Autodesk Fusion 360 part; units mm, degrees
sketch "Sketch1" plane through (0, 0, 0) normal (0, 0, 1) x (1, 0, 0)
  line L0 (0, 44) -> (67, 44)
  line L1 (67, -44) -> (0, -44)
  line L2 (0, 0) -> (67, 0) construction
  line L3 (0, 44) -> (0, -44)
  line L4 (80.435, -13.435) -> (49.8701, -44)
  line L5 (80.435, 13.435) -> (49.8701, 44)
  arc A0 (80.435, -13.435) -> (80.435, 13.435) centre (67, 0) ccw
  dimension "d2" = 67
  dimension "d3" = 88
  dimension "d4" = 67
  dimension "d6" = 38
  dimension "d9" = 45
  dimension "d10" = 45
extrude "Extrude2" add sketch "Sketch1" along normal blind 10
sketch "Sketch5" plane through (0, 0, 10) normal (0, 0, 1) x (-1, 0, 0)
  line L0 (-49.8701, 44) -> (-80.435, 13.435)
  arc A0 (-80.435, 13.435) -> (-80.435, -13.435) centre (-67, 0) ccw
  line L1 (-80.435, -13.435) -> (-49.8701, -44)
  line L2 (-49.8701, -44) -> (0, -44)
  line L3 (0, -44) -> (0, 44)
  line L4 (0, 44) -> (-49.8701, 44)
  line L5 (0, -44) -> (13, -44)
  line L6 (13, -44) -> (13, -19)
  line L7 (13, -19) -> (19, -19)
  line L8 (19, 0) -> (0, 0) construction
  line L9 (0, 44) -> (13, 44)
  line L10 (13, 44) -> (13, 19)
  line L11 (13, 19) -> (19, 19)
  arc A1 (19, -19) -> (19, 19) centre (19, 0) ccw
  line L12 (0, -19) -> (-3, -19)
  line L13 (-3, -19) -> (-3, -5)
  line L14 (-3, -5) -> (-7, -5)
  line L15 (-7, -5) -> (-7, 0)
  line L16 (0, 19) -> (-3, 19)
  line L17 (-3, 19) -> (-3, 5)
  line L18 (-3, 5) -> (-7, 5)
  line L19 (-7, 5) -> (-7, 0)
  line L20 (0, -44) -> (0, -19)
  line L21 (0, 19) -> (0, 44)
  dimension "d15" = 13
  dimension "d16" = 38
  dimension "d17" = 6
  dimension "d18" = 3
  dimension "d19" = 14
  dimension "d20" = 4
extrude "Extrude4" add sketch "Sketch5" along normal blind 40 contours L3 L12 L13 L14 L15 L16 L17 L18 L19
extrude "Extrude3" add sketch "Sketch5" along normal blind 40 and the other way blind 10 contours L3 L5 L6 L7 L9 L10 L11 A1 L20 L21
ref_plane "WorkPlane1" through (18.435, 0, 25) normal (0, 1, 0) x (-1, 0, 0)
sketch "Sketch7" plane through (7, 0, 0) normal (1, 0, 0) x (0, 1, 0)
  line L0 (-5, 10) -> (5, 10)
  line L1 (5, 10) -> (5, 50)
  line L2 (5, 50) -> (-5, 50)
  line L3 (-5, 50) -> (-5, 10)
  line L4 (0, 50) -> (0, 10) construction
sketch "Sketch8" plane through (0, 0, 10) normal (0, 0, 1) x (-1, 0, 0)
  line L0 (-47, 36) -> (-47, -54) construction
  line L1 (-47, -9) -> (-3.8729, -9) construction
  line L2 (-47, -9) -> (-47, -34) construction
  line L3 (-47, -9) -> (-11, -9) construction
  line L4 (-67, 44) -> (-67, -44) construction
  line L5 (-67, -9) -> (-67, -34) construction
  line L6 (-67, -9) -> (-31, -9) construction
  line L7 (-67, 0) -> (-7.0889, 0) construction
  line L8 (-31, 0) -> (-31, -25) construction
  line L9 (-31, 0) -> (-31, 25) construction
  point P0 (-67, 44)
  point P1 (-67, -44)
  dimension "d37" = 25
  dimension "d39" = 36
  dimension "d45" = 25
  dimension "d49" = 25
sketch "Sketch6" plane through (18.435, 0, 25) normal (0, 1, 0) x (1, 0, 0)
  line L0 (-11.435, 15) -> (-11.435, -25)
  line L1 (-11.435, -25) -> (48.565, 15)
  line L2 (48.565, 15) -> (-11.435, 15)
  point P0 (-11.435, 15)
  point P1 (-11.435, -25)
  point P2 (48.565, 15)
extrude "Extrude6" add sketch "Sketch6" along normal mid plane 10
hole "Hole2" at (-19, 0, 50) direction (0, 0, -1) diameter 19 depth 50 tip angle 118
hole "Hole3" at (31, 25, 10) direction (0, 0, -1) diameter 10 depth 50 tip angle 118
hole "Hole4" at (31, -25, 10) direction (0, 0, -1) diameter 10 depth 50 tip angle 118
fillet "Fillet7" radius 13 2 edges at (49.8701, -44, 5) (49.8701, 44, 5)
fillet "Fillet8" radius 3 2 edges at (0, 19, 30) (0, -19, 30)
fillet "Fillet9" radius 6 2 edges at (-13, -19, 25) (-13, 19, 25)
extrude "Extrude5" [suppressed]
fillet "Fillet3" [suppressed]
fillet "Fillet4" [suppressed]
fillet "Fillet5" [suppressed]
fillet "Fillet6" [suppressed]
sketch "Sketch9" plane through (0, 0, 50) normal (0, 0, 1) x (-1, 0, 0)
  line L0 (-3, 19) -> (-3, 5)
  line L1 (-3, 5) -> (-7, 5)
  line L2 (-7, -5) -> (-3, -5)
  line L3 (-3, -5) -> (-3, -19)
  arc A0 (0, -22) -> (-3, -19) centre (-3, -22) ccw
  line L4 (0, -22) -> (0, -44)
  line L5 (0, -44) -> (13, -44)
  line L6 (13, -44) -> (13, -25)
  arc A1 (19, -19) -> (13, -25) centre (19, -25) ccw
  arc A2 (19, -19) -> (19, 19) centre (19, 0) ccw
  arc A3 (13, 25) -> (19, 19) centre (19, 25) ccw
  line L7 (13, 25) -> (13, 44)
  line L8 (13, 44) -> (0, 44)
  line L9 (0, 44) -> (0, 22)
  arc A4 (-3, 19) -> (0, 22) centre (-3, 22) ccw
  circle A5 centre (19, 0) radius 9.5 construction
  line L10 (-7, 5) -> (-7, 0)
  line L11 (-7, 0) -> (-7, -5)
  dimension "d33" = 19
hole "Hole1" [suppressed]
Read the model definition and answer for the solid it produces. Units are mm, in the model's axes. A direction names the side the tool comes from. Give positions to 0.01 mm unless a question says otherwise; leave off trailing zeros. Write each loop counter-clockwise with the first axis right and the second up, starting at its lowest first coordinate (ties: lowest second). Pieces come first, ordered by that corner, then holes. Notation, with made-up numbers: (-39, 82.25) - (-4, 82.25) arc R21 cw to (-4, 120.25) - close; hole circle Ø3 at (72.25, -11). An arc over 180 degrees is marked (long way). Answer in a Markdown table with one row per item. Add a question column.
Item 1: A tool of negligible diameter and unlimited length cuts with its end or side. For faces 1 (the face through (3, -44, 8)), 2 (the face through (27, 5, 25)), 3 (the face through (-13, -35, 25)), 4 (the face through (33, 10, 10)), from which of +Z, -Z, +X, -X, +Y, -Y can it reach the whole face along a straight path? Write none if from no direction.
Item 2: Find the intervals of material crossed by L1, parallel to Y at x = 31, z = 5.75; L2, parallel to Y at x = -19, z = 15.5; L3, parallel to Z at x = 51, y = 23, in increasing order.
Item 3: Section D-D, the plane x = 31 is taken. Write down the section's boundary in (y, z), and give its area (3 significant figures).
Item 4: Section C-C, the plane x = -15 is taken. Write down the section's boundary in (y, z), and give its area (3 significant figures).
Item 5: Determine the mould class of faces 5 (the face through (31, 30, 5)), 6 (the face through (-13, 35, 25)), 7 (the face through (49.39, -43.04, 5.07)) for opening direction X: pulls with the +X half, pulls with the -X half, needs draft (parallel to the pull), parting line crosses it, or undercut.
Item 6: Flat-ended cylindrical pins translate along their axes: P1, Ø5, axis at x = 15.5, z = 39, coming from the +Y side; P2, Ø2, axis at y = 18, z = 17, coming from the +X side; P3, Ø11, axis at y = -30, z = 31.5, coming from the +X side; P4, Ø1, axis at x = -15, y = 34, coming from the -Z side. Find the tip coordinate at first contact, or state that the pin passes through.
Item 7: Section A-A, the plane y = 0 is taken. Write down the section's boundary in (x, z).
Recorded:
| question | item | result |
|---|---|---|
| 1 | face 1 | +Z, -Z, +X, -X, -Y |
| 1 | face 2 | +Z, +X, +Y |
| 1 | face 3 | +Z, -Z, -X, -Y |
| 1 | face 4 | +Z, +X |
| 2 | L1 | y = -44 to -30, -20 to 20, 30 to 44 |
| 2 | L2 | y = -19 to -9.5, 9.5 to 19 |
| 2 | L3 | z = 0 to 10 |
| 3 | outline | (-44, 0) - (-30, 0) - (-30, 10) - (-44, 10) - close; (-20, 0) - (20, 0) - (20, 10) - (5, 10) - (5, 34) - (-5, 34) - (-5, 10) - (-20, 10) - close; (30, 0) - (44, 0) - (44, 10) - (30, 10) - close |
| 3 | area | 920 mm2 |
| 4 | outline | (-20.53, 0) - (-8.62, 0) - (-8.62, 50) - (-20.53, 50) - close; (8.62, 0) - (20.53, 0) - (20.53, 50) - (8.62, 50) - close |
| 4 | area | 1,190 mm2 |
| 5 | face 5 | undercut |
| 5 | face 6 | pulls with the -X half |
| 5 | face 7 | pulls with the +X half |
| 6 | P1 | stops at y = 5 |
| 6 | P2 | stops at x = 3 |
| 6 | P3 | stops at x = 0 |
| 6 | P4 | passes through |
| 7 | outline | (-38, 0) - (-28.5, 0) - (-28.5, 50) - (-38, 50) - close; (-9.5, 0) - (86, 0) - (86, 10) - (67, 10) - (7, 50) - (-9.5, 50) - close |
